Input: part model. Units: mm. Frame: model coordinates. Face numbers are marked on the shaded views. A direction names the side the tool comes from. Coordinates: 2 decimals unless noted, no trailing zeros. Order: outer loops, then holes, each group sorted by start corner. A loop starts at its lowest first (then second) coordinate and runs counter-clockwise, first axis right, second up.
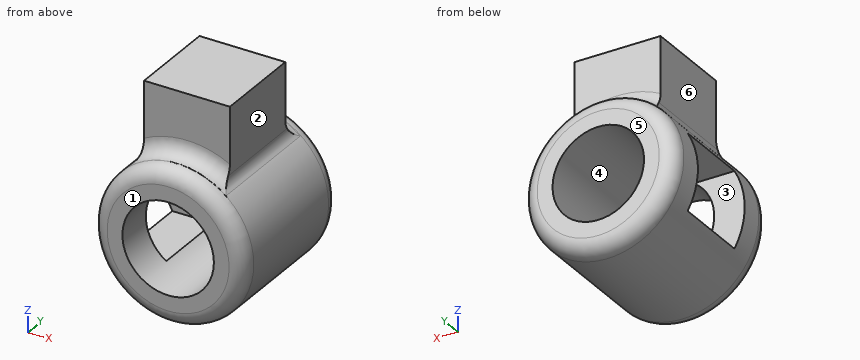
from build123d import *

# Parameters (mm, degrees)
F0_R     = 25
F0_R_2   = 15
F1_DEPTH = 50
F2_W     = 25
F2_H     = 25
F3_DEPTH = 25
F5_R     = 5
F6_W     = 28.14582
F6_H     = 29.589206
F7_DEPTH = 25
F8_R     = 5


with BuildPart() as f1:
    # F0 (on Front) → F1 (new body)
    with BuildSketch(Plane.XZ):
        Circle(F0_R)
        Circle(F0_R_2, mode=Mode.SUBTRACT)
    extrude(amount=F1_DEPTH)

    # F2 (on Right) → F3 (cut)
    with BuildSketch(Plane.YZ):
        with Locations((-25, 0)):
            Rectangle(F2_W, F2_H)
    extrude(amount=-F3_DEPTH, mode=Mode.SUBTRACT)

    # F5
    f5_edges = [f1.edges().sort_by_distance(p)[0] for p in [
        (-25, -50, 0),
        (-25, 0, 0),
    ]]
    fillet(f5_edges, radius=F5_R)

    # F6 (on offset) → F7 (join)
    with BuildSketch(Plane.XY.offset(20)):
        with Locations((0, -25.138795)):
            Rectangle(F6_W, F6_H)
    extrude(amount=F7_DEPTH)

    # F8
    f8_edges = [f1.edges().sort_by_distance(p)[0] for p in [
        (-14.07291, -25.138795, 20.662846),
        (0, -10.344192, 25),
        (14.07291, -25.138795, 20.662846),
        (0, -39.933398, 25),
    ]]
    fillet(f8_edges, radius=F8_R)


solid = f1.part
Item 1: Pin query (flat end, axial travel): pin 1 Ø14.5 at (x, y) = (-15.5, -30.5) entering from -Z; pin 2 Ø24 at (y, z) = (-25.5, 32) entering from -X; pin 3 Ø5 at (y, z) = (-5.5, 8) entering from +X. Return the tip coordinate at first contact, or that it passes through.
Response values:
pin 1: stops at z = -23.6
pin 2: stops at x = -15.2
pin 3: stops at x = 24.39
Item 2: Cut plane B-B on x = 0. Return loops of the section in (y, z), then the cut area to 3 significant figures.
Response values:
outline: (-50, -20) arc R5 ccw to (-45, -25) - (-5, -25) arc R5 ccw to (0, -20) - (0, -15) - (-50, -15) - close; (-50, 15) - (0, 15) - (0, 20) arc R5 ccw to (-5, 25) - (-5.34, 25) arc R5 cw to (-10.34, 30) - (-10.34, 45) - (-39.93, 45) - (-39.93, 30) arc R5 cw to (-44.93, 25) - (-45, 25) arc R5 ccw to (-50, 20) - close
area: 1,580 mm2
Item 3: Cut plane C-C on y = -24. Return loops of the section in (x, z).
Response values:
outline: (-21.65, -12.5) arc R25 ccw (long way) to (15.89, 19.3) arc R5 cw to (14.07, 23.16) - (14.07, 45) - (-14.07, 45) - (-14.07, 23.16) arc R5 cw to (-15.89, 19.3) arc R25 ccw to (-21.65, 12.5) - (-8.29, 12.5) arc R15 cw (long way) to (-8.29, -12.5) - close
Item 4: Cut plane D-D on y = -42.5. Return loops of the section in (x, z).
Response values:
outline: (-15.89, 19.3) arc R25 ccw (long way) to (15.89, 19.3) arc R5 cw to (14.5, 21.14) arc R25.63 ccw to (-14.5, 21.14) arc R5 cw to start; hole circle Ø30 at (0, 0)
Item 5: Draft query along X for the marked faces 4, 5 and 6. Return one class per face: pulls with the +X half, pulls with the -X half, needs draft (parallel to the pull), parting line crosses it, or undercut.
Response values:
face 4: undercut
face 5: needs draft
face 6: pulls with the -X half
Item 6: Cut plane A-A on z = 0. Return loops of the section in (x, y).
Response values:
outline: (-25, -45) arc R5 ccw to (-20, -50) - (-15, -50) - (-15, -37.5) - (-25, -37.5) - close; (-25, -12.5) - (-15, -12.5) - (-15, 0) - (-20, 0) arc R5 ccw to (-25, -5) - close; (15, -50) - (20, -50) arc R5 ccw to (25, -45) - (25, -5) arc R5 ccw to (20, 0) - (15, 0) - close
Item 7: Ray query, probe 1 along Z at (x, y) = (0, -25.5); probe 2 along Y at (x, z) = (-5.5, 31); probe 3 along X at (y, z) = (-21, 32). Return the intervals inside material, ascending.
Response values:
probe 1: z = -25 to -15, 15 to 45
probe 2: y = -39.93 to -10.34
probe 3: x = -14.07 to 14.07
Item 8: Access query for the marked faces 1, 2 and 3. Directions: +Z, -Z, +X, -X, +Y, -Y. A direction counts if a zero-diameter tool reaches every point of the face in a straight line with its end or side. Return the directions, or none.
Response values:
face 1: +Z, -Z, +X, -X, -Y
face 2: +Z, +X, +Y, -Y
face 3: -X
